```python
from build123d import *

# Parameters (mm, degrees)
F0_W     = 48
F0_H     = 48
F1_DEPTH = 6
F2_R     = 21
F3_DEPTH = 10
F4_R     = 3.2
F4_R_2   = 1.35
F5_DEPTH = 12
F6_R     = 3
F7_DEPTH = 16.001


with BuildPart() as f1:
    # F0 (on Top) → F1 (new body)
    with BuildSketch(Plane.XY):
        Rectangle(F0_W, F0_H)
    extrude(amount=F1_DEPTH)

    # F2 (on face) → F3 (join)
    with BuildSketch(Plane.XY.offset(6)):
        Circle(F2_R)
    extrude(amount=F3_DEPTH)

    # F4 (on face) → F5 (cut)
    with BuildSketch(Plane.XY.offset(16)):
        with Locations((-14, 0)):
            Circle(F4_R)
        with Locations((14, 0)):
            Circle(F4_R)
        with Locations((-8, 4.75)):
            Circle(F4_R_2)
        with Locations((8, 4.75)):
            Circle(F4_R_2)
        with Locations((-8, -4.75)):
            Circle(F4_R_2)
        with Locations((8, -4.75)):
            Circle(F4_R_2)
    extrude(amount=-F5_DEPTH, mode=Mode.SUBTRACT)

    # F6 (on face) → F7 (cut, through all)
    with BuildSketch(Plane.XY.offset(16)):
        with Locations((0, -14)):
            Circle(F6_R)
    extrude(amount=-F7_DEPTH, mode=Mode.SUBTRACT)


solid = f1.part
```
Geometry check sheet. Reference: the model listing, model coordinates, mm. A direction names the side the tool comes from. Coordinates: 2 decimals unless noted, no trailing zeros. Write each loop counter-clockwise with the first axis right and the second up, starting at its lowest first coordinate (ties: lowest second). Pieces come first, ordered by that corner, then holes. Notation, with made-up numbers: M 32,60.25 L 68,60.25 A20 ccw 68,66.25 Z; hole C 85.5,-12 d3. An arc over 180 degrees is marked long. Use one line per item in the form item = value. Start each with the question number.
1) Thickness scan on probe 1 along X at (y, z) = (2, 15); probe 2 along X at (y, z) = (-1.5, 15); probe 3 along Y at (x, z) = (8, 7). Record the ranges inside material, lowest first. Write a range as from..to.
2) Set-up check for faces 1 (the flat face through (0, 0, 0)), 2 (the flat face through (-22, 0, 6)): record each of +Z, -Z, +X, -X, +Y, -Y from which the full face is reachable in a straight line by a thin tool's end or side.
3) Section check B-B on z = 13.25. Enter the section's corners in (x, y).
4) Section check D-D on x = 14.5. Enter the section's corners in (y, z).
5) Release check for a two-part mould opening along Y. For faces 3 (the flat face through (0, 0, 16)), 4 (the flat face through (0, 24, 3)), 5 (the flat face through (8, 5, 4)), 6 (the flat face through (-8, -5, 4)) record: pulls with the +Y half, pulls with the -Y half, needs draft (parallel to the pull), parting line crosses it, or undercut.
6) Section check A-A on y = 0. Enter the section's corners in (x, z), and give its area (3 significant figures).
7) Section check C-C on y = -13. Enter the section's corners in (x, z), and give its area (3 significant figures).
8) Go/stop test with flat-tipped pins: pin 1 Ø0.8 at (x, y) = (-7.5, -4.5) entering from +Z; pin 2 Ø1 at (y, z) = (0, 9.5) entering from +X; pin 3 Ø1 at (x, z) = (-1, 13.5) entering from +Y. Record where each tip stops, or that it passes through.
Responses:
q1.probe_1 = -20.9..-16.5, -11.5..11.5, 16.5..20.9
q1.probe_2 = -20.95..-16.83, -11.17..11.17, 16.83..20.95
q1.probe_3 = -19.42..-6.1, -3.4..3.4, 6.1..19.42
q2.face_1 = -Z, +X, -X, +Y, -Y
q2.face_2 = +Z
q3.outline = C 0,0 d42; hole C -14,0 d6.4; hole C -8,-4.75 d2.7; hole C -8,4.75 d2.7; hole C 0,-14 d6; hole C 8,-4.75 d2.7; hole C 8,4.75 d2.7; hole C 14,0 d6.4
q4.outline = M -24,0 L 24,0 L 24,6 L 15.19,6 L 15.19,16 L 3.16,16 L 3.16,4 L -3.16,4 L -3.16,16 L -15.19,16 L -15.19,6 L -24,6 Z
q5.face_3 = needs draft
q5.face_4 = pulls with the +Y half
q5.face_5 = undercut
q5.face_6 = undercut
q6.outline = M -24,0 L 24,0 L 24,6 L 21,6 L 21,16 L 17.2,16 L 17.2,4 L 10.8,4 L 10.8,16 L -10.8,16 L -10.8,4 L -17.2,4 L -17.2,16 L -21,16 L -21,6 L -24,6 Z
q6.area = 554 mm2
q7.outline = M -24,0 L -2.83,0 L -2.83,16 L -16.49,16 L -16.49,6 L -24,6 Z; M 2.83,0 L 24,0 L 24,6 L 16.49,6 L 16.49,16 L 2.83,16 Z
q7.area = 527 mm2
q8.pin_1 = 4
q8.pin_2 = 21
q8.pin_3 = 20.99
